CAD build for the part. Positions are in the model's coordinates, mm. A direction names the side the tool comes from. Coordinates: 2 decimals unless noted, no trailing zeros. Write each loop counter-clockwise with the first axis right and the second up, starting at its lowest first coordinate (ties: lowest second). Pieces come first, ordered by that corner, then holes. Notation, with made-up numbers: (-16, 11) - (-4, 11) arc R28 ccw to (-4, 43) - close; hole circle Ø2 at (4, 33.25). An arc over 180 degrees is marked (long way). One line per question, with ' | ' between items. Start each with the question number.
1. Band-saw the part on C-C, the plane x = 34. Write the cut outline in (y, z).
2. Probe line 1 (Y direction, x = 114.5, z = 3); line 2 (X direction, y = 125.5, z = 2); line 3 (X direction, y = 1, z = 204.5). List the from-to ranges inside material, lowest first.
3. Which spindle directions (+Z, -Z, +X, -X, +Y, -Y) get a long thin tool onto all of the face, cutting with end or side? Do faces 1 (the flat face through (-2, 10, -5)), 2 (the flat face through (10, 5, 2)), 3 (the flat face through (0, 0, 260)), 4 (the flat face through (-10, 0, 0)), 5 (the cylindrical face through (-1.08, -4.88, 133.25)). Say none if no direction does.
4. Band-saw the part on A-A, the plane y = 0. Write the cut outline in (x, z), then the cut area to 3 significant figures.
from build123d import *

# Parameters (mm, degrees)
SKETCH1_W           = 20
SKETCH1_H           = 20
BOSS_EXTRUDE1_DEPTH = 10
SKETCH2_R           = 5
BOSS_EXTRUDE2_DEPTH = 250
SKETCH3_R           = 5
BOSS_EXTRUDE3_DEPTH = 250
SKETCH4_R           = 5
BOSS_EXTRUDE4_DEPTH = 250


with BuildPart() as part:
    # Sketch1 → Boss-Extrude1 (new, symmetric)
    with BuildSketch(Plane(origin=(0, 0, 0), x_dir=(1, 0, 0), z_dir=(0, 1, 0))):
        Rectangle(SKETCH1_W, SKETCH1_H)
    extrude(amount=BOSS_EXTRUDE1_DEPTH, both=True)

    # Sketch2 → Boss-Extrude2 (add)
    with BuildSketch(Plane(origin=(10, 0, 0), x_dir=(0, 0, -1), z_dir=(1, 0, 0))):
        Circle(SKETCH2_R)
    extrude(amount=BOSS_EXTRUDE2_DEPTH)

    # Sketch3 → Boss-Extrude3 (add)
    with BuildSketch(Plane.XY.offset(10)):
        Circle(SKETCH3_R)
    extrude(amount=BOSS_EXTRUDE3_DEPTH)

    # Sketch4 → Boss-Extrude4 (add)
    with BuildSketch(Plane(origin=(0, 10, 0), x_dir=(1, 0, 0), z_dir=(0, 1, 0))):
        with Locations(Location((0, 0, 0), (0, 0, 270))):
            Circle(SKETCH4_R)
    extrude(amount=BOSS_EXTRUDE4_DEPTH)


solid = part.part
Filled in:
1) outline: circle Ø10 at (0, 0)
2) line 1: y = -4 to 4 | line 2: x = -4.58 to 4.58 | line 3: x = -4.9 to 4.9
3) face 1: +Y | face 2: +X | face 3: +Z, +X, -X, +Y, -Y | face 4: +Z, -Z, -X, +Y, -Y | face 5: +Z
4) outline: (-10, -10) - (10, -10) - (10, -5) - (260, -5) - (260, 5) - (10, 5) - (10, 10) - (5, 10) - (5, 260) - (-5, 260) - (-5, 10) - (-10, 10) - close | area: 5,400 mm²
